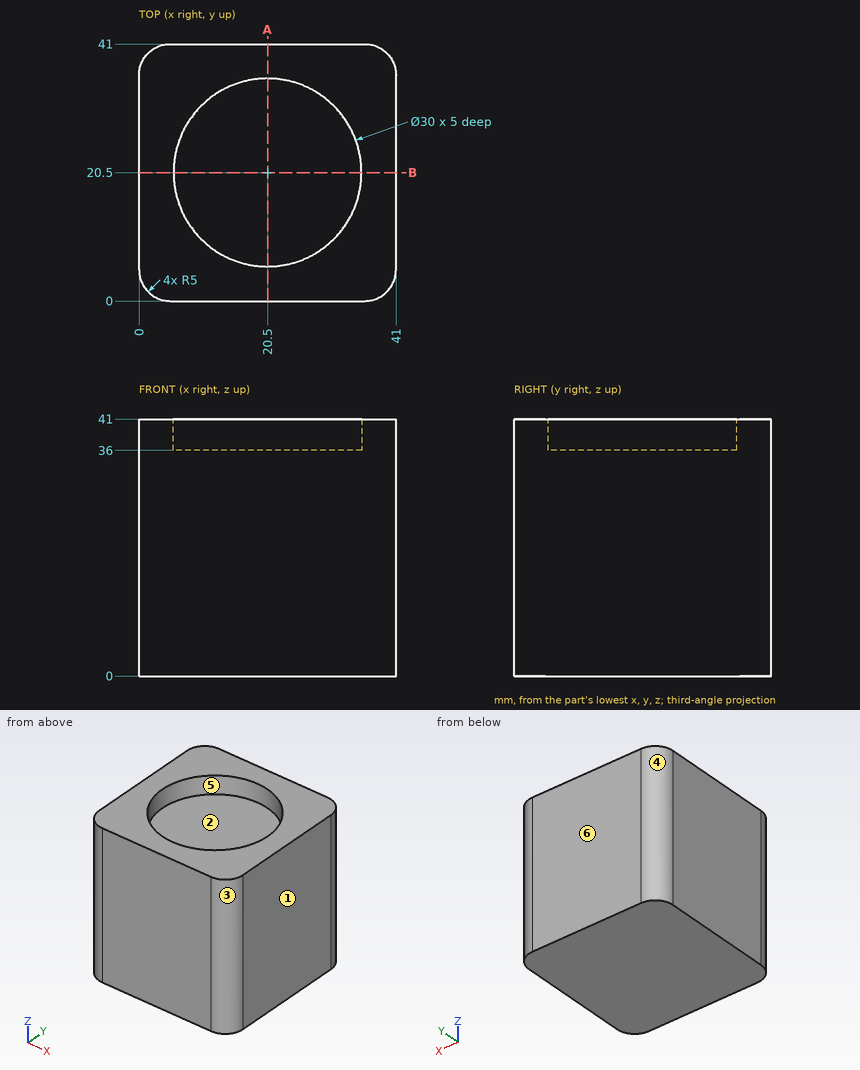
Part print with two shaded views. Sizes in mm from the minimum x, y, z corner. A direction names the side the tool comes from. Round coordinates to 2 decimals unless told otherwise and drop trailing zeros. Loops run counter-clockwise (first coordinate to the right, second up) from the corner with the lowest first, then second, coordinate; pieces in that order, holes last. Notation, with made-up numbers: M 68.5,50.25 L 103.5,50.25 A18 ccw 103.5,76.25 Z; hole C -37,-23.75 d6. An arc over 180 degrees is marked long. Put each result on its own line as item: value. Start each with the question number.
Item 1: Drill centre lines: line 1 along Y through (x, z) = (20.5, 39.3); line 2 along X through (y, z) = (20, 39); line 3 along Z through (x, y) = (14.5, 19). Where is each one in solid material? Low to high.
Item 2: Cut at A-A (x = 20.5). List the corners of the cut face in (y, z).
Item 3: Mould opens along X. For the marked faces 3, 4, 5 and 6 say: released by +X, released by -X, zero draft, split by the parting line, or undercut.
Item 4: 3-axis set-ups, long thin cutter, end or side, ignore diameter. For the marked faces 1 and 2: which of +Z, -Z, +X, -X, +Y, -Y reach the whole face in a straight line?
Answer block:
1. line 1: 0 to 5.5, 35.5 to 41
1. line 2: 0 to 5.51, 35.49 to 41
1. line 3: 0 to 36
2. outline: M 0,0 L 41,0 L 41,41 L 35.5,41 L 35.5,36 L 5.5,36 L 5.5,41 L 0,41 Z
3. face 3: released by +X
3. face 4: released by -X
3. face 5: undercut
3. face 6: zero draft
4. face 1: +Z, -Z, +X, +Y, -Y
4. face 2: +Z
